Could you check a few things on this model? Use its own coordinates, in mm. Give positions to 0.01 mm unless a question says otherwise; leave off trailing zeros. Order: outer loops, then holes, each group sorted by start corner. A loop starts at its lowest first (then second) coordinate and runs counter-clockwise, first axis right, second up. Notation, with made-up numbers: (79.5, 66.5) - (128.5, 66.5) arc R20 ccw to (128.5, 93.5) - close; hole circle Ø7 at (77.5, -7.75). An arc over 180 degrees is marked (long way). Put each result on its own line as item: value.
from build123d import *

# Parameters (mm, degrees)
CUT_EXTRUDE_1_DEPTH = 2


with BuildPart() as part:
    # ｽｹｯﾁ1 → 回転1 (revolve)
    with BuildSketch(Plane.XY):
        Polygon((-4, 0), (-4, 2.0095), (-3.5095, 2.5), (-0.75, 2.5), (0, 1.75), (0, 0), align=None)
    revolve(axis=Axis((0, 0, 0), (-1, 0, 0)))

    # ｽｹｯﾁ2 → ｶｯﾄ - 押し出し1 (cut)
    with BuildSketch(Plane.ZY.offset(4)):
        Polygon((0.721687836, -1.25), (1.443375673, 0), (0.721687836, 1.25), (-0.721687836, 1.25), (-1.443375673, 0), (-0.721687836, -1.25), align=None)
    extrude(amount=-CUT_EXTRUDE_1_DEPTH, mode=Mode.SUBTRACT)

    # ｽｹｯﾁ3 → ｶｯﾄ - 回転1 (revolve, cut)
    with BuildSketch(Plane.XY):
        Polygon((-2, 0), (-2, 1.25), (-1.278312164, 0), align=None)
    revolve(axis=Axis((-1.278312164, 0, 0), (-1, 0, 0)), mode=Mode.SUBTRACT)


solid = part.part
1) Suppose I cut it at B-B, the plane x = -0.55. List the corners of the cut face in (y, z) for me, and give its area (3 significant figures).
Filled in:
outline: circle Ø4.6 at (0, 0)
area: 16.6 mm^2
2) Suppose I cut it at A-A, the plane x = -2.55. List the corners of the cut face in (y, z) for me, and give its area (3 significant figures).
Filled in:
outline: circle Ø5 at (0, 0); hole (-1.25, -0.72) - (0, -1.44) - (1.25, -0.72) - (1.25, 0.72) - (0, 1.44) - (-1.25, 0.72) - close
area: 14.2 mm^2
3) Suppose I cut it at C-C, the plane x = -1.35. List the corners of the cut face in (y, z) for me.
Filled in:
outline: circle Ø5 at (0, 0); hole circle Ø0.25 at (0, 0)
4) If I drill on line 1 (Y direction, x = -2.5, z = -0.05); line 2 (Y direction, x = -2.95, z = -0.9); line 3 (Z direction, x = -3.8, y = -1), over which ranges is the centre line in solid material (lowest first)? Write a range as [from, to].
Filled in:
line 1: y = [-2.5, -1.25], [1.25, 2.5]
line 2: y = [-2.33, -0.94], [0.94, 2.33]
line 3: z = [-1.97, -0.87], [0.87, 1.97]
5) I'm going to push flat-ended pins straight in: pin 1 (1 mm diameter, centred on y = -0.5, z = 0.5, fed in from -X); pin 2 (1 mm diameter, centred on x = -1, y = 1, fed in from +Z); pin 3 (1 mm diameter, centred on x = -3, z = -2, fed in from +Y). Where does each tip first touch, or does it pass through?
Filled in:
pin 1: stops at x = -1.98
pin 2: stops at z = 2.45
pin 3: stops at y = 2
6) We'd pull the mould along Y, two halves only. Please class faces 1 (the flat face through (-3.014, -0.616, -1.088)), 2 (the flat face through (0, 0, 0)), 3 (the cylindrical face through (-2.11, -0.54, 2.44)): pulls with the +Y half, pulls with the -Y half, needs draft (parallel to the pull), parting line crosses it, or undercut.
Filled in:
face 1: undercut
face 2: needs draft
face 3: parting line crosses it
